Check sheet for the modelled part. Datum: model origin and axes. Units: mm. Face numbers are marked on the shaded views. Give positions to 0.01 mm unless a question says otherwise; leave off trailing zeros. Write each loop counter-clockwise with the first axis right and the second up, starting at its lowest first coordinate (ties: lowest second). Pieces come first, ordered by that corner, then holes. Notation, with made-up numbers: M 84,57 L 99,57 A20 ccw 99,66 Z; hole C 68,5.5 d5. An arc over 180 degrees is marked long. Use CSV: the item, a comma, the result in double quotes. Start each with the question number.
1. Scan lines: line 1 (X direction, y = -238, z = 8.75); line 2 (X direction, y = -198, z = 8); line 3 (Y direction, x = 39, z = 1). Record each from-to range of solid material in increasing order.
2. Cross-section at B-B, the plane z = 8.5. State how many separate pieces and enclosed holes the cut face has, and give its area (3 significant figures).
3. Cross-section at A-A, the plane y = -196. Enter the section's corners in (x, z), and give its area (3 significant figures).
4. Depth check by flat-ended pin: P1, Ø5, axis at y = -192, z = 6, coming from the +X side; P2, Ø2.5, axis at x = 54.45, y = -258.43, coming from the -Z side; P3, Ø4.5, axis at y = -171.5, z = 5.5, coming from the +X side; P4, Ø2, axis at x = -50.5, z = 3.5, coming from the -Y side. Enter the tip coordinate at first touch or a pass-through.
5. Cross-section at D-D, the plane x = 8.5. Enter the section's corners in (y, z).
6. Cross-section at C-C, the plane x = -59.5. Enter the section's corners in (y, z), and give its area (3 significant figures).
7. Mould release check, pull along X, two halves, no side actions. Record for the marked faces 1, 2 and 3: +X half, -X half, draft (parallel to the pull), parting line (faces both ways), or undercut.
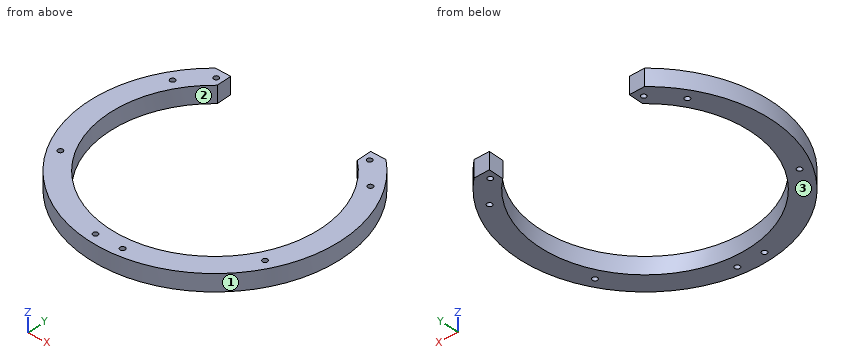
from build123d import *

# Parameters (mm, degrees)
RESSALTO_EXTRUS_O1_DEPTH = 10
ESBO_O2_R                = 1.5
CORTE_EXTRUS_O1_DEPTH    = 10
ESBO_O3_W                = 82
ESBO_O3_H                = 21.575786581
CORTE_EXTRUS_O2_DEPTH    = 11


with BuildPart() as part:
    # Esboço1 → Ressalto-extrusão1 (new body)
    with BuildSketch(Plane.XY):
        with BuildLine():
            Line((44.495405461, -168.430491325), (22.44625518, -168.430491325))
            ThreePointArc((22.44625518, -168.430491325), (-5.504594539, -286.832190763), (-33.455444258, -168.430491325))
            Line((-33.455444258, -168.430491325), (-55.504594539, -168.430491325))
            ThreePointArc((-55.504594539, -168.430491325), (-5.504594539, -299.332190763), (44.495405461, -168.430491325))
        make_face()
    extrude(amount=RESSALTO_EXTRUS_O1_DEPTH)

    # Esboço2 → Corte-extrusão1 (cut)
    with BuildSketch(Plane.XY.offset(10)):
        with Locations((39.44625518, -173.430491325)):
            Circle(ESBO_O2_R)
        with Locations((52.44625518, -187.430491325)):
            Circle(ESBO_O2_R)
        with Locations((54.44625518, -258.430491325)):
            Circle(ESBO_O2_R)
        with Locations((-13.455444258, -293.430491325)):
            Circle(ESBO_O2_R)
        with Locations((2.44625518, -293.430491325)):
            Circle(ESBO_O2_R)
        with Locations((-65.455444258, -258.430491325)):
            Circle(ESBO_O2_R)
        with Locations((-63.455444258, -187.430491325)):
            Circle(ESBO_O2_R)
        with Locations((-50.455444258, -173.430491325)):
            Circle(ESBO_O2_R)
    extrude(amount=-CORTE_EXTRUS_O1_DEPTH, mode=Mode.SUBTRACT)

    # Esboço3 → Corte-extrusão2 (cut, through all)
    with BuildSketch(Plane.XY.offset(10)):
        with Locations((-5.504594539, -170.044523075)):
            Rectangle(ESBO_O3_W, ESBO_O3_H)
    extrude(amount=-CORTE_EXTRUS_O2_DEPTH, mode=Mode.SUBTRACT)


solid = part.part
Worked answers:
1,line 1,"x = -79.25 to -66.49, 55.48 to 68.24"
1,line 2,"x = -75.73 to -62.19, 51.18 to 64.72"
1,line 3,"y = -284.7 to -268.21, -180.45 to -174.86, -172 to -168.43"
2,separate pieces,"1"
2,enclosed holes,"8"
2,area,"4,180 mm^2"
3,outline,"M -74.95,0 L -61.21,0 L -61.21,10 L -74.95,10 Z; M 50.2,0 L 63.94,0 L 63.94,10 L 50.2,10 Z"
3,area,"275 mm^2"
4,P1,"stops at x = 63.31"
4,P2,"passes through"
4,P3,"stops at x = 49.87"
4,P4,"stops at y = -285.07"
5,outline,"M -298.01,0 L -285.24,0 L -285.24,10 L -298.01,10 Z"
6,outline,"M -276.39,0 L -255.81,0 L -255.81,10 L -276.39,10 Z; M -192.86,0 L -172.28,0 L -172.28,10 L -192.86,10 Z"
6,area,"412 mm^2"
7,face 1,"parting line"
7,face 2,"undercut"
7,face 3,"draft"
